Check sheet for the drawn part. Datum: minimum x, y, z corner. Units: mm. A direction names the side the tool comes from. Give positions to 0.01 mm unless a question says otherwise; leave off trailing zeros. Order: outer loops, then holes, each group sorted by start corner. A loop starts at its lowest first (then second) coordinate and runs counter-clockwise, first axis right, second up. Notation, with made-up numbers: (-25.75, -25.5) - (-8.75, -25.5) arc R22 ccw to (-8.75, 3.5) - close; hole circle Ø11 at (-10.5, -18). An arc over 180 degrees is marked (long way). Answer as a JSON object with one key per item and string values. Group by question number.
(1) Section check A-A (z = 83). Record the boundary of the cut face in (x, y), then the cut area to 4 significant figures.
(2) Access from +Z, -Z, +X, -X, +Y, -Y to the whole of each face (thin tool, end or side, straight path). Record for the marked faces 1 and 2.
(3) Section check C-C (z = 9.5). Record the boundary of the cut face in (x, y).
(4) Section check D-D (y = 6.25). Record the boundary of the cut face in (x, z).
(5) Thickness scan on line 1 (X direction, y = 0.45, z = 83); line 2 (X direction, y = 12.75, z = 48). Record the ranges inside material, lowest first.
(6) Depth check by flat-ended pin: pin 1 Ø8 at (x, z) = (5, 62.5) entering from -Y; pin 2 Ø4.5 at (x, z) = (6.5, 83) entering from +Y; pin 3 Ø9 at (x, z) = (9.5, 67) entering from +Y; pin 4 Ø1.5 at (y, z) = (15.5, 48) entering from +X. Enter the tip coordinate at first touch or a pass-through.
(7) Section check B-B (x = 6.5). Record the boundary of the cut face in (y, z), then the cut area to 4 significant figures.
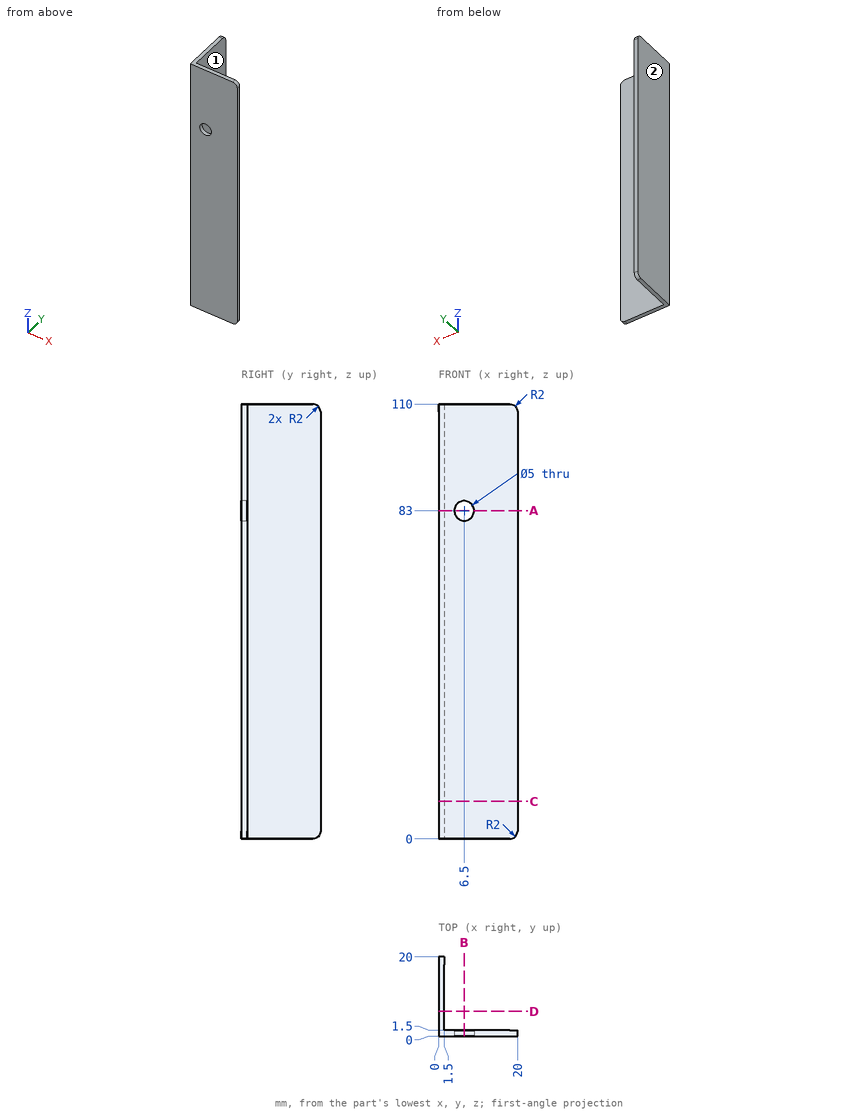
Solutions:
{
 "1": {"outline": "(0, 0) - (4, 0) - (4, 1.5) - (1.5, 1.5) - (1.5, 20) - (0, 20) - close; (9, 0) - (20, 0) - (20, 1.5) - (9, 1.5) - close", "area": "50.25 mm2"},
 "2": {"face 1": "+Z, -Z, +X, +Y", "face 2": "+Z, -Z, -X, +Y, -Y"},
 "3": {"outline": "(0, 0) - (20, 0) - (20, 1.5) - (1.5, 1.5) - (1.5, 20) - (0, 20) - close"},
 "4": {"outline": "(0, 0) - (1.5, 0) - (1.5, 110) - (0, 110) - close"},
 "5": {"line 1": "x = 0 to 4, 9 to 20", "line 2": "x = 0 to 1.5"},
 "6": {"pin 1": "stops at y = 0", "pin 2": "passes through", "pin 3": "stops at y = 1.5", "pin 4": "stops at x = 1.5"},
 "7": {"outline": "(0, 0) - (1.5, 0) - (1.5, 80.5) - (0, 80.5) - close; (0, 85.5) - (1.5, 85.5) - (1.5, 110) - (0, 110) - close", "area": "157.5 mm2"}
}
